```python
from build123d import *

# Parameters (mm, degrees)
SKETCH1_W           = 30
SKETCH1_H           = 75
BOSS_EXTRUDE1_DEPTH = 3.175
SKETCH2_W           = 3.175
SKETCH2_H           = 10
BOSS_EXTRUDE2_DEPTH = 3.175


with BuildPart() as part:
    # Sketch1 → Boss-Extrude1 (new body)
    with BuildSketch(Plane(origin=(0, 0, 0), x_dir=(1, 0, 0), z_dir=(0, 1, 0))):
        Rectangle(SKETCH1_W, SKETCH1_H)
    extrude(amount=BOSS_EXTRUDE1_DEPTH)

    # Sketch2 → Boss-Extrude2 (add)
    with BuildSketch(Plane(origin=(0, 3.175, 0), x_dir=(1, 0, 0), z_dir=(0, 1, 0))):
        with Locations((-16.5875, 0)):
            Rectangle(SKETCH2_W, SKETCH2_H)
        with Locations((-16.5875, -20)):
            Rectangle(SKETCH2_W, SKETCH2_H)
        with Locations((-16.5875, 20)):
            Rectangle(SKETCH2_W, SKETCH2_H)
        with Locations((16.5875, -20)):
            Rectangle(SKETCH2_W, SKETCH2_H)
        with Locations((16.5875, 0)):
            Rectangle(SKETCH2_W, SKETCH2_H)
        with Locations((16.5875, 20)):
            Rectangle(SKETCH2_W, SKETCH2_H)
    extrude(amount=-BOSS_EXTRUDE2_DEPTH)


solid = part.part
```
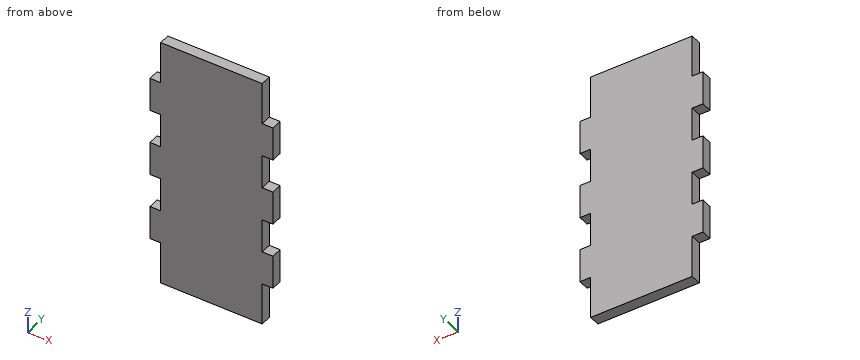
Could you check a few things on this model? Use its own coordinates, in mm. Coordinates: 2 decimals unless noted, no trailing zeros. Order: outer loops, then holes, each group sorted by start corner. A loop starts at its lowest first (then second) coordinate and runs counter-clockwise, first axis right, second up. Notation, with made-up numbers: M -26.75,26.5 L 11.25,26.5 A19 ccw 11.25,36.5 Z; hole C 40.5,33.25 d8. An arc over 180 degrees is marked long. Use one line per item in the form item = value. Start each with the question number.
1. Please list where these lines run through material, in increasing order: line 1 (Z direction, x = 15.5, y = 2.65); line 2 (X direction, y = 1.45, z = -7).
2. Suppose I cut it at A-A on y = 0.75. Write out the boundary of the cut face in (x, z) (3 decimals).
3. For pin 1 (1.6 mm diameter, centred on y = 1.5, z = -28.5, fed in from +X); pin 2 (1 mm diameter, centred on y = 1.5, z = -31.5, fed in from -X); pin 3 (1.6 mm diameter, centred on x = 16.5, y = 2, fed in from +Z), each with a flat end and sliding along its axis, tell me the tip position at first contact or that it passes through.
4. Suppose I cut it at B-B on z = -29. Write out the boundary of the cut face in (x, y) (3 decimals).
Geometry says:
q1.line_1 = -25 to -15, -5 to 5, 15 to 25
q1.line_2 = -15 to 15
q2.outline = M -18.175,-25 L -15,-25 L -15,-37.5 L 15,-37.5 L 15,-25 L 18.175,-25 L 18.175,-15 L 15,-15 L 15,-5 L 18.175,-5 L 18.175,5 L 15,5 L 15,15 L 18.175,15 L 18.175,25 L 15,25 L 15,37.5 L -15,37.5 L -15,25 L -18.175,25 L -18.175,15 L -15,15 L -15,5 L -18.175,5 L -18.175,-5 L -15,-5 L -15,-15 L -18.175,-15 Z
q3.pin_1 = 15
q3.pin_2 = -15
q3.pin_3 = 25
q4.outline = M -15,0 L 15,0 L 15,3.175 L -15,3.175 Z
